from build123d import *

# Parameters (mm, degrees)
SKETCH2_R                = 7.5
BOSS_EXTRUDE1_DEPTH      = 2.5
BOSS_EXTRUDE2_DEPTH      = 5
BOSS_EXTRUDE2_DEPTH_BACK = 5
SKETCH3_R                = 2.5


with BuildPart() as part:
    # Sketch2 → Boss-Extrude1 (new, symmetric)
    with BuildSketch(Plane.XY):
        Circle(SKETCH2_R)
    extrude(amount=BOSS_EXTRUDE1_DEPTH, both=True)

    # Sketch3 → Boss-Extrude2 (add, two sides: drawn at the far end of the back side and taken through both)
    with BuildSketch(Plane.XY.offset(-BOSS_EXTRUDE2_DEPTH_BACK)):
        Circle(SKETCH3_R)
    extrude(amount=BOSS_EXTRUDE2_DEPTH + BOSS_EXTRUDE2_DEPTH_BACK)


solid = part.part
Verification items for the finished model (mm, model axes). A direction names the side the tool comes from. Round coordinates to 2 decimals unless told otherwise and drop trailing zeros. Loops run counter-clockwise (first coordinate to the right, second up) from the corner with the lowest first, then second, coordinate; pieces in that order, holes last. Notation, with made-up numbers: (7, 85) - (21, 85) arc R26 ccw to (21, 123) - close; hole circle Ø9 at (83.25, 16.25). An arc over 180 degrees is marked (long way). Use a Markdown table: item, result. Add a question column.
1. Section check B-B, the plane x = -2. Record the boundary of the cut face in (y, z), plus the area to 3 significant figures.
2. Section check A-A, the plane y = 0. Record the boundary of the cut face in (x, z), plus the area to 3 significant figures.
3. Gauge pin test, flat ends, axial feed: pin 1 (1 mm diameter, centred on x = 5, y = 2, fed in from -Z); pin 2 (4 mm diameter, centred on y = 5, z = 0.5, fed in from -X); pin 3 (5 mm diameter, centred on x = 5, z = 0.5, fed in from -Y). Record the tip position at first contact, or that the pin passes through.
4. Thickness scan on probe 1 along Z at (x, y) = (0.25, -5); probe 2 along Y at (x, z) = (-0.75, 2); probe 3 along Y at (x, z) = (-4.75, 0.5). Record the ranges inside material, lowest first. Write a range as [from, to].
5. Access from +Z, -Z, +X, -X, +Y, -Y to the whole of each face (thin tool, end or side, straight path). Record for faces 1 (the face through (-0.54, -2.44, 3.73)), 2 (the face through (0, 0, 5)), 3 (the face through (-0.54, -2.44, -3.77)).
6. Section check C-C, the plane z = 3.75. Record the boundary of the cut face in (x, y), plus the area to 3 significant figures.
7. Section check D-D, the plane x = -4.5. Record the boundary of the cut face in (y, z).
Checks:
| question | item | result |
|---|---|---|
| 1 | outline | (-7.23, -2.5) - (-1.5, -2.5) - (-1.5, -5) - (1.5, -5) - (1.5, -2.5) - (7.23, -2.5) - (7.23, 2.5) - (1.5, 2.5) - (1.5, 5) - (-1.5, 5) - (-1.5, 2.5) - (-7.23, 2.5) - close |
| 1 | area | 87.3 mm^2 |
| 2 | outline | (-7.5, -2.5) - (-2.5, -2.5) - (-2.5, -5) - (2.5, -5) - (2.5, -2.5) - (7.5, -2.5) - (7.5, 2.5) - (2.5, 2.5) - (2.5, 5) - (-2.5, 5) - (-2.5, 2.5) - (-7.5, 2.5) - close |
| 2 | area | 100 mm^2 |
| 3 | pin 1 | stops at z = -2.5 |
| 3 | pin 2 | stops at x = -6.87 |
| 3 | pin 3 | stops at y = -7.07 |
| 4 | probe 1 | z = [-2.5, 2.5] |
| 4 | probe 2 | y = [-7.46, 7.46] |
| 4 | probe 3 | y = [-5.8, 5.8] |
| 5 | face 1 | +Z |
| 5 | face 2 | +Z, +X, -X, +Y, -Y |
| 5 | face 3 | -Z |
| 6 | outline | circle Ø5 at (0, 0) |
| 6 | area | 19.6 mm^2 |
| 7 | outline | (-6, -2.5) - (6, -2.5) - (6, 2.5) - (-6, 2.5) - close |
